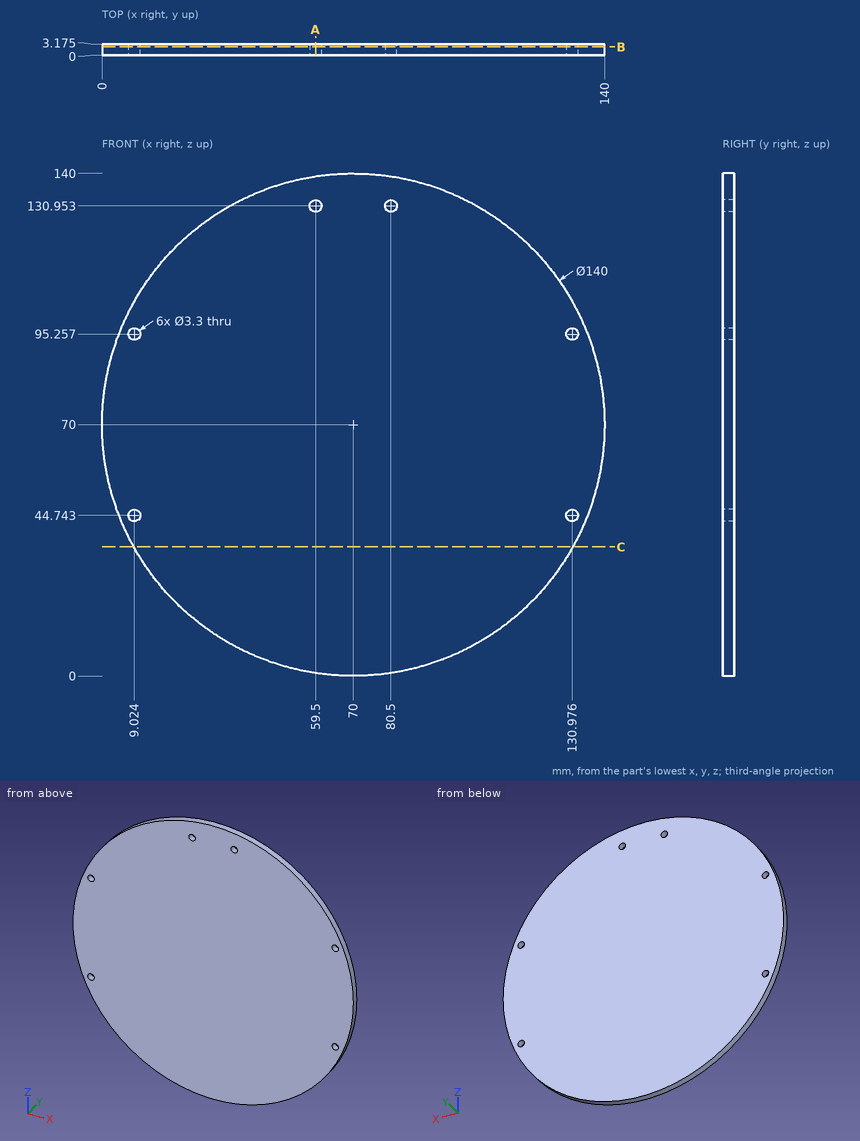
Geometry check sheet. Reference: drawing and pictorial views, mm from the part's lowest x, y, z. Round coordinates to 2 decimals unless told otherwise and drop trailing zeros. Order: outer loops, then holes, each group sorted by start corner. A loop starts at its lowest first (then second) coordinate and runs counter-clockwise, first axis right, second up. Notation, with made-up numbers: M 29,-16.5 L 86,-16.5 A19 cw 86,2.5 Z; hole C 27.25,-8.5 d3. An arc over 180 degrees is marked long. One line per item, written item: value. Start each with the question number.
1. Section check C-C on z = 36. Enter the section's corners in (x, y) (3 decimals).
2. Section check A-A on x = 59.5. Enter the section's corners in (y, z) (3 decimals).
3. Section check B-B on y = 2.35. Enter the section's corners in (x, z).
4. Gauge pin test, flat ends, axial feed: P1, Ø3, axis at x = 130.98, z = 44.74, coming from the -Y side; P2, Ø2, axis at x = 122.5, z = 105.5, coming from the -Y side; P3, Ø1.5, axis at y = 0.5, z = 43, coming from the +X side. Record the tip position at first contact, or that the pin passes through.
5. Scan lines: line 1 along X through (y, z) = (0.85, 94) (1 decimal); line 2 along X through (y, z) = (1.5, 131.5); line 3 along Z through (x, y) = (80.5, 0.65). Record each from-to range of solid material in increasing order.
Results found:
1. outline: M 8.812,0 L 131.188,0 L 131.188,3.175 L 8.812,3.175 Z
2. outline: M 0,0.792 L 3.175,0.792 L 3.175,129.303 L 0,129.303 Z; M 0,132.603 L 3.175,132.603 L 3.175,139.208 L 0,139.208 Z
3. outline: C 70,70 d140; hole C 9.02,44.74 d3.3; hole C 9.02,95.26 d3.3; hole C 59.5,130.95 d3.3; hole C 80.5,130.95 d3.3; hole C 130.98,44.74 d3.3; hole C 130.98,95.26 d3.3
4. P1: through
4. P2: y = 0
4. P3: x = 134.89
5. line 1: 4.2 to 8, 10.1 to 129.9, 132 to 135.8
5. line 2: 36.57 to 57.94, 61.06 to 78.94, 82.06 to 103.43
5. line 3: 0.79 to 129.3, 132.6 to 139.21
